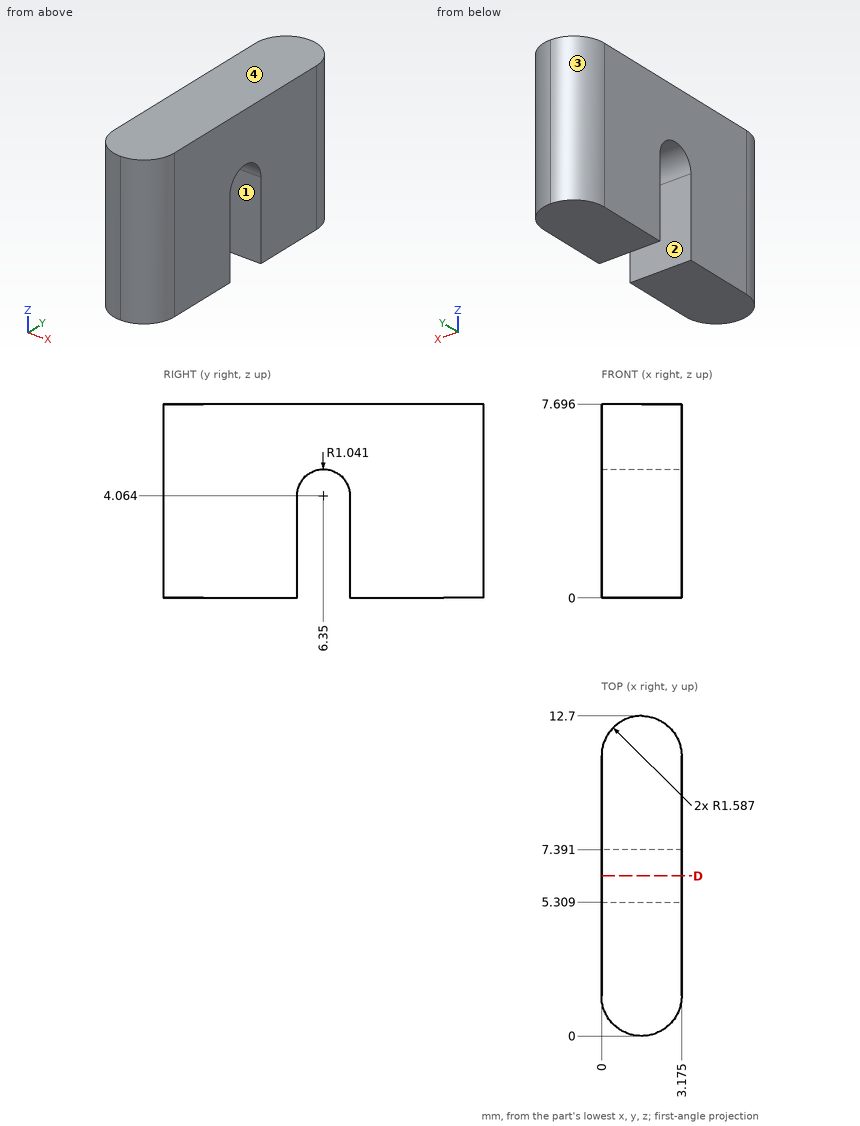
Part print with two shaded views. Sizes in mm from the minimum x, y, z corner. Coordinates: 2 decimals unless noted, no trailing zeros. Write each loop counter-clockwise with the first axis right and the second up, starting at its lowest first coordinate (ties: lowest second). Pieces come first, ordered by that corner, then holes. Notation, with made-up numbers: (70, -13.5) - (89, -13.5) arc R20 ccw to (89, 17.5) - close; hole circle Ø2 at (66, 31). An arc over 180 degrees is marked (long way). One line per item, written item: value. Start each with the question number.
1. Probe line 1 (Y direction, x = 1.55, z = 3.25); line 2 (Y direction, x = 3, z = 4) (1 decimal); line 3 (X direction, y = 1.5, z = 6.5). List the from-to ranges inside material, lowest first. Write a range as from..to.
2. Mould opens along Y. For the marked faces 1, 2, 3 and 4 say: released by +Y, released by -Y, zero draft, split by the parting line, or undercut.
3. Slice it at D-D (y = 6.35). Write the cut outline in (x, z) (1 decimal).
Answers below:
1. line 1: y = 0..5.31, 7.39..12.7
1. line 2: y = 0.9..5.3, 7.4..11.8
1. line 3: x = 0..3.17
2. face 1: undercut
2. face 2: undercut
2. face 3: released by +Y
2. face 4: zero draft
3. outline: (0, 5.1) - (3.2, 5.1) - (3.2, 7.7) - (0, 7.7) - close
